from build123d import *

# Parameters (mm, degrees)
PAD003_DEPTH    = 2
POCKET059_DEPTH = 14


with BuildPart() as part:
    # Sketch161 (on XY_Plane of Origin) → AdditiveLoft001 section 0
    with BuildSketch(Plane.XY):
        with BuildLine():
            ThreePointArc((-8.035319, 4.6), (-16.839863, 0.753527), (-20, -8.32))
            Line((-20, -8.32), (20, -8.32))
            ThreePointArc((20, -8.32), (16.839863, 0.753527), (8.035319, 4.6))
            Line((-8.035319, 4.6), (8.035319, 4.6))
        make_face()
    # Sketch162 (on XY_Plane of Origin) → AdditiveLoft001 section 1
    with BuildSketch(Plane.XY.offset(-10)):
        with BuildLine():
            ThreePointArc((-6, 3), (-11, -2), (-6, -7))
            Line((-6, -7), (6, -7))
            ThreePointArc((6, -7), (11, -2), (6, 3))
            Line((-6, 3), (6, 3))
        make_face()
    loft()

    # Sketch163 (on XZ_Plane of Origin) → Pad003 (new body, symmetric)
    with BuildSketch(Plane.XZ.offset(3)):
        with BuildLine():
            Line((-12, 0), (-12, 6))
            ThreePointArc((-12, 6), (-14.386092, 6.886092), (-13.5, 4.5))
            Line((-13.5, 4.5), (-13.5, 0))
            Line((-13.5, 0), (-12, 0))
        make_face()
        with BuildLine():
            Line((12, 0), (12, 6))
            ThreePointArc((13.5, 4.5), (14.386092, 6.886092), (12, 6))
            Line((13.5, 4.5), (13.5, 0))
            Line((13.5, 0), (12, 0))
        make_face()
    extrude(amount=PAD003_DEPTH, both=True)

    # Sketch164 (on Face14 of Pad003) → Pocket059 (cut)
    with BuildSketch(Plane(origin=(0, 0, -10), x_dir=(1, 0, 0), z_dir=(0, 0, -1))):
        with BuildLine():
            Line((0, 13.5), (2, 13.5))
            Line((2, 5.5), (2, 13.5))
            ThreePointArc((-2, 5.5), (0, 1.5), (2, 5.5))
            Line((-2, 13.5), (-2, 5.5))
            Line((0, 13.5), (-2, 13.5))
        make_face()
    extrude(amount=-POCKET059_DEPTH, mode=Mode.SUBTRACT)


with BuildPart() as part_1:
    # Body placement: moved
    add(part.part.moved(Location((0, 0, -106))))


solid = part_1.part
Source: CAD feature listing. Evaluate the final solid. Frame: model axes, mm. A direction names the side the tool comes from. Round coordinates to 2 decimals unless told otherwise and drop trailing zeros. Loops run counter-clockwise (first coordinate to the right, second up) from the corner with the lowest first, then second, coordinate; pieces in that order, holes last. Notation, with made-up numbers: M 33,-13 L 54,-13 A16 ccw 54,0 Z; hole C -22.5,41.5 d10. An arc over 180 degrees is marked long. Return JSON: item names as keys, results as strings. Group by question number.
1. Section query A-A on z = -103. Output: boundary loops of the cut face in (x, y).
2. Material intervals for line 1 along Z through (x, y) = (5, -5.25); line 2 along X through (y, z) = (-4, -109); line 3 along X through (y, z) = (-4, -108.75), sorted ascending. Write a range as from..to.
3. Mould query, pull axis Z, two halves, no side actions, for faces 1 (the face through (-12, -3, -103)), 2 (the face through (0, -1, -116)), 3 (the face through (14.42, -3.03, -99.15)). Classes: released by +Z, released by -Z, zero draft, split by the parting line, or undercut.
4. Reachability of faces 4 (the face through (13, -5, -102)), 5 (the face through (-13.5, -3, -104)), 6 (the face through (13.5, -3, -104)) from +Z, -Z, +X, -X, +Y, -Y: full face, straight path, thin tool, end or side. Return the list, or none.
5. Pin query (flat end, axial travel): pin 1 (1.4 mm diameter, centred on x = -13.5, z = -103, fed in from +Y); pin 2 (6.5 mm diameter, centred on x = -5.5, y = -1, fed in from +Z); pin 3 (3 mm diameter, centred on x = -13, z = -102, fed in from -Y); pin 4 (6.5 mm diameter, centred on x = 0, y = -4, fed in from -Z). Return the tip coordinate at first contact, or that it passes through.
Checks:
{
 "1": {"outline": "M -13.5,-5 L -12,-5 L -12,-1 L -13.5,-1 Z; M 12,-5 L 13.5,-5 L 13.5,-1 L 12,-1 Z"},
 "2": {"line 1": "z = -116..-106", "line 2": "x = -16.41..-2.5, 2.5..16.41", "line 3": "x = -16.66..-2.5, 2.5..16.66"},
 "3": {"face 1": "zero draft", "face 2": "released by -Z", "face 3": "undercut"},
 "4": {"face 4": "+Z, +X, -X, -Y", "face 5": "-X, +Y, -Y", "face 6": "+X, +Y, -Y"},
 "5": {"pin 1": "stops at y = -1", "pin 2": "stops at z = -106", "pin 3": "stops at y = -5", "pin 4": "stops at z = -116"}
}
